Autodesk Inventor part; units mm, degrees
ref_plane "YZ Plane" through (0, 0, 0) normal (1, 0, 0) x (0, 1, 0)
ref_plane "XZ Plane" through (0, 0, 0) normal (0, 1, 0) x (-1, 0, 0)
ref_plane "XY Plane" through (0, 0, 0) normal (0, 0, 1) x (1, 0, 0)
sketch "Sketch1" plane through (0, 0, 0) normal (0, 0, 1) x (1, 0, 0)
  circle A0 centre (0, 0) radius 20
  circle A1 centre (0, 0) radius 25 construction
  circle A2 centre (0, 0) radius 32
  circle A3 centre (0, 25) radius 3.25
  circle A4 centre (-25, 0) radius 3.25
  circle A5 centre (0, -25) radius 3.25
  circle A6 centre (25, 0) radius 3.25
  dimension "d1" = 50
  dimension "d0" = 40
  dimension "d2" = 64
  dimension "d3" = 6.5
  dimension "d6" = 360
extrude "Extrusion1" add sketch "Sketch1" along normal blind 0.5
properties part number "CylinderPacking"
Input: part model. Units: mm. Frame: model coordinates. Give positions to 0.01 mm unless a question says otherwise; leave off trailing zeros. Order: outer loops, then holes, each group sorted by start corner. A loop starts at its lowest first (then second) coordinate and runs counter-clockwise, first axis right, second up. Notation, with made-up numbers: (84.5, -31) - (143.5, -31) arc R23 ccw to (143.5, -12) - close; hole circle Ø10 at (-15.5, 89). An arc over 180 degrees is marked (long way). Put each result on its own line as item: value.
Item 1: Section query B-B, the plane z = 0.15. Return loops of the section in (x, y), then the cut area to 3 significant figures.
Found:
outline: circle Ø64 at (0, 0); hole circle Ø6.5 at (-25, 0); hole circle Ø40 at (0, 0); hole circle Ø6.5 at (0, -25); hole circle Ø6.5 at (0, 25); hole circle Ø6.5 at (25, 0)
area: 1,830 mm^2
Item 2: Section query D-D, the plane x = 25. Return loops of the section in (y, z).
Found:
outline: (-19.97, 0) - (-3.25, 0) - (-3.25, 0.5) - (-19.97, 0.5) - close; (3.25, 0) - (19.97, 0) - (19.97, 0.5) - (3.25, 0.5) - close
Item 3: Draft query along Y for faces 1 (the cylindrical face through (-4.336, 19.524, 0.246)), 2 (the flat face through (14, 15, 0.5)), 3 (the cylindrical face through (-6.94, 31.24, 0.25)). Return one class per face: +Y half, -Y half, draft (parallel to the pull), parting line (faces both ways), or undercut.
Found:
face 1: undercut
face 2: draft
face 3: parting line
Item 4: Section query C-C, the plane y = 26. Return loops of the section in (x, z), then the cut area to 3 significant figures.
Found:
outline: (-18.65, 0) - (-3.09, 0) - (-3.09, 0.5) - (-18.65, 0.5) - close; (3.09, 0) - (18.65, 0) - (18.65, 0.5) - (3.09, 0.5) - close
area: 15.6 mm^2
Item 5: Ray query, L1, parallel to Y at x = 0, z = 0.2; L2, parallel to X at y = -16, z = 0.2; L3, parallel to X at y = 8, z = 0.35. Return the intervals inside material, ascending. Write a range as from..to.
Found:
L1: y = -32..-28.25, -21.75..-20, 20..21.75, 28.25..32
L2: x = -27.71..-12, 12..27.71
L3: x = -30.98..-18.33, 18.33..30.98
Item 6: Section query A-A, the plane x = 0. Return loops of the section in (y, z).
Found:
outline: (-32, 0) - (-28.25, 0) - (-28.25, 0.5) - (-32, 0.5) - close; (-21.75, 0) - (-20, 0) - (-20, 0.5) - (-21.75, 0.5) - close; (20, 0) - (21.75, 0) - (21.75, 0.5) - (20, 0.5) - close; (28.25, 0) - (32, 0) - (32, 0.5) - (28.25, 0.5) - close
Item 7: Contact query for a flat-ended pin moving along its axis: pin 1 (7.5 mm diameter, centred on x = 25, y = 0, fed in from -Z). Output: stop coordinate, or through.
Found:
pin 1: stops at z = 0
